from build123d import *

# Parameters (mm, degrees)
F0_R            = 42.2899684473
F1_DEPTH        = 6.35
F3_DEPTH        = 6.351
F3_COPIES_COUNT = 12
F5_DEPTH        = 6.351


# Not quite as in the source:
# - a pattern or mirror of a feature is missing from the dataset's text; its kind, count and spacing are read off the source's solid


with BuildPart() as f1:
    # F0 (on Front) → F1 (new body)
    with BuildSketch(Plane.XZ):
        Circle(F0_R)
    extrude(amount=-F1_DEPTH)

    # F2 (on face) → F3 (cut, through all)
    with BuildSketch(Plane.XZ):
        with BuildLine():
            ThreePointArc((-41.4371280171, -8.4501983983), (-39.9301176937, -6.1715058408), (-37.4314860419, -5.0668068974))
            ThreePointArc((-37.4314860419, -5.0668068974), (-37.42798385, -5.0663435871), (-37.4244819792, -5.065877856))
            ThreePointArc((-37.4244819792, -5.065877856), (-32.9892827736, 0.0035327048), (-37.4314860419, 5.0668068974))
            ThreePointArc((-37.4314860419, 5.0668068974), (-39.9301176937, 6.1715058408), (-41.4371280171, 8.4501983983))
            ThreePointArc((-41.4371280171, 8.4501983983), (-42.2899684473, 0), (-41.4371280171, -8.4501983983))
        make_face()
    f3 = extrude(amount=-F3_DEPTH, mode=Mode.SUBTRACT)

    # F3_copies: F3 ×12 about axis
    f3_copies_axis = Axis((0, 0, 0), (0, 1, 0))
    for i in range(1, F3_COPIES_COUNT):
        add(f3.rotate(f3_copies_axis, i * 360 / F3_COPIES_COUNT), mode=Mode.SUBTRACT)

    # F4 (on face) → F5 (cut, through all)
    with BuildSketch(Plane.XZ):
        Polygon((0.8374305792, 6.3609167663), (-5.0900002214, 3.9056945387), (-5.9274308006, -2.4552222276), (-0.8374305792, -6.3609167663), (5.0900002214, -3.9056945387), (5.9274308006, 2.4552222276), align=None)
    extrude(amount=-F5_DEPTH, mode=Mode.SUBTRACT)


solid = f1.part
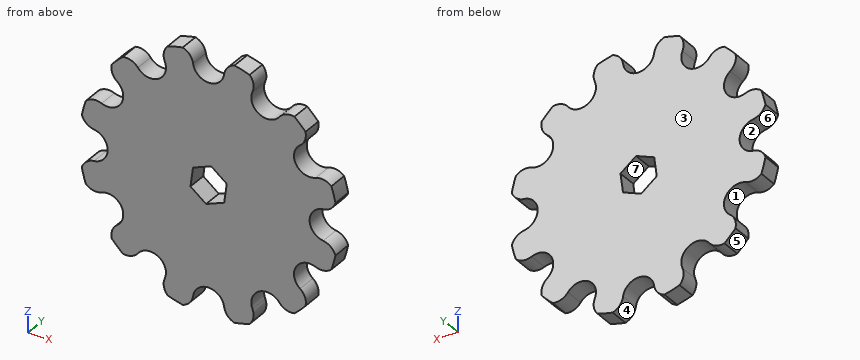
Could you check a few things on this model? Use its own coordinates, in mm. Face numbers are marked on the shaded views. A direction names the side the tool comes from. Round coordinates to 2 decimals unless told otherwise and drop trailing zeros. Loops run counter-clockwise (first coordinate to the right, second up) from the corner with the lowest first, then second, coordinate; pieces in that order, holes last. Notation, with made-up numbers: (-28, -12) -> (26, -12) arc R29 cw to (26, 18) -> close; hole circle Ø4 at (83.25, 8.25). An arc over 180 degrees is marked (long way). Use CSV: the item, a comma, the result in double quotes.
(1) Suppose I cut it at C-C on x = -7. Write out the boundary of the cut face in (y, z), plus the area to 3 significant figures.
Return value:
outline,"(0, -40.71) -> (6.35, -40.71) -> (6.35, 40.71) -> (0, 40.71) -> close"
area,"517 mm²"
(2) If I drill on probe 1 along X at (y, z) = (5, -29.5); probe 2 along Z at (x, y) = (19, 6); probe 3 along X at (y, z) = (4.25, 2.5), over which ranges is the centre line in solid material (lowest first)? Write a range as [from, to].
Return value:
probe 1,"x = [-30.3, -22.78], [-15.32, 15.32], [22.78, 30.3]"
probe 2,"z = [-27.89, 27.89]"
probe 3,"x = [-33.64, -5.28], [5.87, 33.64]"
(3) Suppose I cut it at A-A on x = 34. Write out the boundary of the cut face in (y, z), plus the area to 3 significant figures.
Return value:
outline,"(0, -14.04) -> (6.35, -14.04) -> (6.35, -3.05) -> (0, -3.05) -> close; (0, 3.05) -> (6.35, 3.05) -> (6.35, 14.04) -> (0, 14.04) -> close"
area,"140 mm²"
(4) Will these pins go through, and if not, where does the flat tip stop? pin 1 Ø12 at (x, z) = (25.5, -17.5) entering from -Y; pin 2 Ø1 at (y, z) = (5, 7.5) entering from +X; pin 3 Ø3 at (y, z) = (4.5, -18) entering from -X; pin 4 Ø3 at (y, z) = (2, 21) entering from +X.
Return value:
pin 1,"stops at y = 0"
pin 2,"stops at x = 41.27"
pin 3,"stops at x = -28.57"
pin 4,"stops at x = 29.23"
(5) If we mould it in two halves opening along X, with no side actions, what happens to the marked faces 1, 2 and 3? For each: +X half, -X half, draft (parallel to the pull), parting line (faces both ways), or undercut.
Return value:
face 1,"undercut"
face 2,"-X half"
face 3,"draft"
(6) Suppose I cut it at B-B on x = 20.5. Write out the boundary of the cut face in (y, z), plus the area to 3 significant figures.
Return value:
outline,"(0, -28.09) -> (6.35, -28.09) -> (6.35, 28.09) -> (0, 28.09) -> close"
area,"357 mm²"
(7) For the marked faces 4, 5, 6 and 7, which set-ups out of +Z, -Z, +X, -X, +Y, -Y let a thin tool reach every point of the face, with its end or its side?
Return value:
face 4,"-Z, +Y, -Y"
face 5,"-Z, -X, +Y, -Y"
face 6,"-X, +Y, -Y"
face 7,"+Y, -Y"
